```python
from build123d import *

# Parameters (mm, degrees)
F0_R     = 7.5
F1_DEPTH = 150
F3_DEPTH = 12.5
F4_W     = 25
F4_H     = 20
F5_DEPTH = 36
F6_R     = 6.5
F7_DEPTH = 136


with BuildPart() as f1:
    # F0 (on Right) → F1 (new body)
    with BuildSketch(Plane.YZ):
        Circle(F0_R)
    extrude(amount=F1_DEPTH)

    # F2 (on Front) → F3 (intersect, symmetric)
    with BuildSketch(Plane.XZ):
        Polygon((134.290012, -11.203319), (151.53335, 9.346492), (-5.394438, 11.139952), (-5.394438, -11.203319), align=None)
    extrude(amount=F3_DEPTH, both=True, mode=Mode.INTERSECT)

    # F4 (on Top) → F5 (cut)
    with BuildSketch(Plane.XY):
        with Locations((119.331561, 0.248567)):
            Rectangle(F4_W, F4_H)
    extrude(amount=F5_DEPTH, mode=Mode.SUBTRACT)

    # F6 (on Right) → F7 (cut)
    with BuildSketch(Plane.YZ):
        Circle(F6_R)
    extrude(amount=F7_DEPTH, mode=Mode.SUBTRACT)


solid = f1.part
```
Can you work these out from the model? Positions are in its coordinate system, mm. A direction names the side the tool comes from. Round coordinates to 2 decimals unless told otherwise and drop trailing zeros. Loops run counter-clockwise (first coordinate to the right, second up) from the corner with the lowest first, then second, coordinate; pieces in that order, holes last. Notation, with made-up numbers: M -3.75,75 L 33.25,75 A31 cw 33.25,113 Z; hole C 77.25,-16 d1. An arc over 180 degrees is marked long. Answer in a Markdown table with one row per item.
1. I'm going to push flat-ended pins straight in: pin 1 Ø1 at (x, z) = (59.5, -1) entering from -Y; pin 2 Ø8 at (y, z) = (0, 0) entering from -X; pin 3 Ø4 at (x, z) = (90.5, -5.5) entering from +Y. Where does each tip first touch, or does it pass through?
Established:
| item | result |
|---|---|
| pin 1 | y = -7.48 |
| pin 2 | x = 136 |
| pin 3 | y = 6.63 |
2. If we section it at D-D, the plane x = 115.5: Please give me the cut outline in (y, z), plus the area to 3 significant figures.
Established:
| item | result |
|---|---|
| outline | M -7.5,0 A7.5 ccw 7.5,0 L 6.5,0 A6.5 cw -6.5,0 Z |
| area | 22.0 mm² |
3. On a 3-axis mill with a long thin cutter (end or side, diameter ignored), from which of +Z, -Z, +X, -X, +Y, -Y can I reach the whole of each face in a straight line? I mean faces 5 (the face through (0, -6, 3)), 6 (the face through (106.832, 0, 7)). Say none if no direction works.
Established:
| item | result |
|---|---|
| face 5 | +Z, -Z, -X, +Y, -Y |
| face 6 | +Z, +Y, -Y |
4. If we section it at C-C, the plane x = 38: Please give me the cut outline in (y, z), plus the area to 3 significant figures.
Established:
| item | result |
|---|---|
| outline | C 0,0 d15; hole C 0,0 d13 |
| area | 44.0 mm² |
5. Thinking about a two-plate mould opening in Y: for faces 1 (the face through (136, 0, 0)), 2 (the face through (131.832, 0, 7)), 3 (the face through (67.048, -1.409, -6.345)), 4 (the face through (57.277, 3.461, -6.654)), which applies, pulls with the +Y half, pulls with the -Y half, needs draft (parallel to the pull), parting line crosses it, or undercut?
Established:
| item | result |
|---|---|
| face 1 | undercut |
| face 2 | needs draft |
| face 3 | undercut |
| face 4 | parting line crosses it |
6. If we section it at A-A, the plane y = 0: Please give me the cut outline in (x, z).
Established:
| item | result |
|---|---|
| outline | M 0,-7.5 L 137.4,-7.5 L 149.98,7.5 L 131.83,7.5 L 131.83,6.5 L 136,6.5 L 136,-6.5 L 0,-6.5 Z; M 0,6.5 L 106.83,6.5 L 106.83,7.5 L 0,7.5 Z |
7. Please list where these lines run through material, in increasing order: line 1 (Y direction, x = 106, z = 0); line 2 (Z direction, x = 86.5, y = -2.25). Write a range as from..to.
Established:
| item | result |
|---|---|
| line 1 | -7.5..-6.5, 6.5..7.5 |
| line 2 | -7.15..-6.1, 6.1..7.15 |
8. If we section it at B-B, the plane z = 1.5: Please give me the cut outline in (x, y), plus the area to 3 significant figures.
Established:
| item | result |
|---|---|
| outline | M 0,-7.35 L 106.83,-7.35 L 106.83,-6.32 L 0,-6.32 Z; M 0,6.32 L 106.83,6.32 L 106.83,7.35 L 0,7.35 Z; M 131.83,-7.35 L 144.95,-7.35 L 144.95,7.35 L 131.83,7.35 L 131.83,6.32 L 136,6.32 L 136,-6.32 L 131.83,-6.32 Z |
| area | 359 mm² |
